from build123d import *

# Parameters (mm, degrees)
F0_W      = 96
F0_H      = 64
F1_DEPTH  = 16
F2_W      = 16
F2_H      = 64
F3_DEPTH  = 48
F4_R      = 32
F5_W      = 40
F5_H      = 42
F6_DEPTH  = 28
F8_DEPTH  = 52.07
F9_W      = 40
F9_H      = 12
F10_DEPTH = 28
F12_DEPTH = 25.4
F14_W     = 19.9191475213
F14_H     = 15.9830040127
F15_DEPTH = 25
F17_DEPTH = 25


with BuildPart() as f1:
    # F0 (on Top) → F1 (new body)
    with BuildSketch(Plane.XY):
        with Locations((4.9427039921, 10.6956655151)):
            Rectangle(F0_W, F0_H)
    extrude(amount=F1_DEPTH)

    # F2 (on face) → F3 (join)
    with BuildSketch(Plane.XY.offset(16)):
        with Locations((-35.0572960079, 10.6956655151)):
            Rectangle(F2_W, F2_H)
    extrude(amount=F3_DEPTH)

    # F4
    f4_edges = [f1.edges().sort_by_distance(p)[0] for p in [
        (-35.057296, -21.304334, 64),
    ]]
    fillet(f4_edges, radius=F4_R)

    # F5 (on face) → F6 (join)
    with BuildSketch(Plane.XY.offset(16)):
        with Locations((-7.0572960079, 21.6956655151)):
            Rectangle(F5_W, F5_H)
    extrude(amount=F6_DEPTH)

    # F7 (on face) → F8 (cut)
    with BuildSketch(Plane.XZ.offset(-0.6956655151)):
        with BuildLine():
            ThreePointArc((-19.0572960079, 44), (-7.0572960079, 32), (4.9427039921, 44))
            Line((4.9427039921, 44), (-19.0572960079, 44))
        make_face()
    extrude(amount=-F8_DEPTH, mode=Mode.SUBTRACT)

    # F9 (on face) → F10 (join)
    with BuildSketch(Plane.XY.offset(16)):
        with Locations((32.9427039921, 36.6956655151)):
            Rectangle(F9_W, F9_H)
    extrude(amount=F10_DEPTH)

    # F11 (on face) → F12 (cut)
    with BuildSketch(Plane.XZ.offset(-30.6956655151)):
        Polygon((52.9427039921, 44), (12.9427039921, 44), (52.9427039921, 16), align=None)
    extrude(amount=-F12_DEPTH, mode=Mode.SUBTRACT)

    # F14 (on face) → F15 (cut)
    with BuildSketch(Plane.XY.offset(16)):
        with Locations((42.9831302315, 2.765810062)):
            Rectangle(F14_W, F14_H)
    extrude(amount=-F15_DEPTH, mode=Mode.SUBTRACT)

    # F16 (on face) → F17 (cut)
    with BuildSketch(Plane.XY.offset(16)):
        with BuildLine():
            Line((33.0235564709, 10.7573120683), (33.4770667325, 10.7573120683))
            ThreePointArc((33.4770667325, 10.7573120683), (25.1183803566, 3.0327593017), (32.9427039921, -5.2326089915))
            Line((32.9427039921, -5.2326089915), (32.9427039921, -5.2256919444))
            Line((32.9427039921, -5.2256919444), (33.0235564709, -5.2256919444))
            Line((33.0235564709, -5.2256919444), (33.0235564709, 10.7573120683))
        make_face()
    extrude(amount=-F17_DEPTH, mode=Mode.SUBTRACT)


solid = f1.part
Geometry check sheet. Reference: the model listing, model coordinates, mm. A direction names the side the tool comes from. Round coordinates to 2 decimals unless told otherwise and drop trailing zeros. Loops run counter-clockwise (first coordinate to the right, second up) from the corner with the lowest first, then second, coordinate; pieces in that order, holes last. Notation, with made-up numbers: (-40, 72.25) - (-9, 72.25) arc R24 ccw to (-9, 94.25) - close; hole circle Ø6 at (66.25, 0). An arc over 180 degrees is marked (long way). One line per question, with ' | ' between items. Start each with the question number.
1. Cross-section at D-D on z = 22.5. Record the cut outline in (x, y), then the cut area to 3 significant figures.
2. Tool access check on faces 1 (the face through (52.943, -13, 8)), 2 (the face through (12.943, 15, 30)), 3 (the face through (-23, 22, 44)), 4 (the face through (43, 10.757, 8)). Record the directions out of +Z, -Z, +X, -X, +Y, -Y that give a thin tool (end or side, any length) a straight path to the whole face; none if there is none.
3. Draft check along Y on faces 5 (the face through (9, 22, 44)), 6 (the face through (-6, 42.696, 24)), 7 (the face through (-6, -21.304, 12)), 8 (the face through (43, -5.226, 8)). Enter one of: released by +Y, released by -Y, zero draft, split by the parting line, or undercut.
4. Scan lines: line 1 (Y direction, x = 36.5, z = 11.5); line 2 (Z direction, x = 43, y = 12); line 3 (Y direction, x = 41, z = 22). Record each from-to range of solid material in increasing order. Write a range as [from, to].
5. Cross-section at A-A on x = 42.5. Record the cut outline in (y, z).
6. Cross-section at C-C on x = 7.5. Record the cut outline in (y, z), then the cut area to 3 significant figures.
7. Depth check by flat-ended pin: pin 1 (22.5 mm diameter, centred on x = 33, z = 28, fed in from -Y); pin 2 (6 mm diameter, centred on x = -12.5, y = 3, fed in from +Z); pin 3 (9 mm diameter, centred on x = 10.5, y = 17.5, fed in from +Z). Enter the tip coordinate at first touch or a pass-through.
8. Cross-section at B-B on y = 12. Record the cut outline in (x, z), then the cut area to 3 significant figures.
Taken from the geometry:
1) outline: (-43.06, -21.3) - (-27.06, -21.3) - (-27.06, 0.7) - (12.94, 0.7) - (12.94, 30.7) - (43.66, 30.7) - (43.66, 42.7) - (-43.06, 42.7) - close | area: 3,070 mm²
2) face 1: +Z, -Z, +X, +Y, -Y | face 2: +Z, +X, -Y | face 3: +Z, +X, +Y, -Y | face 4: +Z, -Z, +X
3) face 5: zero draft | face 6: released by +Y | face 7: released by -Y | face 8: undercut
4) line 1: [-21.3, -5.23], [10.76, 42.7] | line 2: [0, 16] | line 3: [30.7, 42.7]
5) outline: (-21.3, 0) - (-5.23, 0) - (-5.23, 16) - (-21.3, 16) - close; (10.76, 0) - (42.7, 0) - (42.7, 23.31) - (30.7, 23.31) - (30.7, 16) - (10.76, 16) - close
6) outline: (-21.3, 0) - (42.7, 0) - (42.7, 44) - (0.7, 44) - (0.7, 16) - (-21.3, 16) - close | area: 2,200 mm²
7) pin 1: y = 30.7 | pin 2: z = 35.47 | pin 3: z = 44
8) outline: (-43.06, 0) - (52.94, 0) - (52.94, 16) - (12.94, 16) - (12.94, 44) - (4.94, 44) arc R12 cw to (-19.06, 44) - (-27.06, 44) - (-27.06, 64) - (-43.06, 64) - close | area: 3,200 mm²
